Autodesk Fusion 360 part; units mm, degrees
sketch "Sketch1" plane through (0, 0, 0) normal (1, 0, 0) x (0, 1, 0)
sketch "Sketch2" plane through (0, 0, 0) normal (0, 0, 1) x (1, 0, 0)
sketch "Sketch3" plane through (0, 0, 0) normal (1, 0, 0) x (0, 1, 0)
sketch "Sketch4" plane through (0, 0, 0) normal (1, 0, 0) x (0, 1, 0)
sketch "Sketch5" plane through (0, 0, 0) normal (0, 1, 0) x (1, 0, 0)
  circle A0 centre (0, 0) radius 18
  circle A1 centre (0, 0) radius 8
  line L0 (0, 11.547) -> (-10, 5.7735)
  line L1 (-10, 5.7735) -> (-10, -5.7735)
  line L2 (-10, -5.7735) -> (0, -11.547)
  line L3 (0, -11.547) -> (10, -5.7735)
  line L4 (10, -5.7735) -> (10, 5.7735)
  line L5 (10, 5.7735) -> (0, 11.547)
  arc A2 (18.3848, -24.0416) -> (24.0416, -18.3848) centre (21.2132, -21.2132) ccw
  arc A3 (-18.3848, 24.0416) -> (-24.0416, 18.3848) centre (-21.2132, 21.2132) ccw
  line L6 (-21.2132, 21.2132) -> (21.2132, -21.2132) construction
  circle A4 centre (21.2132, -21.2132) radius 2
  circle A5 centre (-21.2132, 21.2132) radius 2
  arc A6 (24.0416, 18.3848) -> (18.3848, 24.0416) centre (21.2132, 21.2132) ccw
  arc A7 (-24.0416, -18.3848) -> (-18.3848, -24.0416) centre (-21.2132, -21.2132) ccw
  circle A8 centre (-21.2132, -21.2132) radius 2
  circle A9 centre (21.2132, 21.2132) radius 2
  arc A10 (24.0416, -24.0416) -> (24.0416, 24.0416) centre (0, 0) ccw
  arc A11 (24.0416, 24.0416) -> (-24.0416, 24.0416) centre (0, 0) ccw
  arc A12 (-24.0416, 24.0416) -> (-24.0416, -24.0416) centre (0, 0) ccw
  arc A13 (-24.0416, -24.0416) -> (24.0416, -24.0416) centre (0, 0) ccw
  line L7 (-24.0416, -18.3848) -> (-15.2381, -9.5812)
  line L8 (-21.2132, -21.2132) -> (-12.7279, -12.7279) construction
  line L9 (-9.5812, -15.2381) -> (-18.3848, -24.0416)
  line L10 (9.5812, -15.2381) -> (18.3848, -24.0416)
  line L11 (24.0416, -18.3848) -> (15.2381, -9.5812)
  line L12 (24.0416, 18.3848) -> (15.2381, 9.5812)
  line L13 (12.7279, 12.7279) -> (21.2132, 21.2132) construction
  line L14 (9.5812, 15.2381) -> (18.3848, 24.0416)
  line L15 (-9.5812, 15.2381) -> (-18.3848, 24.0416)
  line L16 (-24.0416, 18.3848) -> (-15.2381, 9.5812)
  line L17 (0, 0) -> (5.6569, 0) construction
  line L18 (8, 0) -> (30, 0) construction
  dimension "d3" = 36
  dimension "d4" = 16
  dimension "d5" = 10
  dimension "d8" = 8
  dimension "d9" = 45
  dimension "d10" = 4
  dimension "d11" = 4
  dimension "d12" = 60
  dimension "d14" = 34
  dimension "d16" = 360
sketch "Sketch6" plane through (0, 0, 0) normal (0, 1, 0) x (1, 0, 0)
extrude "Extrude1" add sketch "Sketch5" along normal blind 10 contours A0 | A0 A2 A6 A10 L11 L12 | A0 A6 L12 L14 | A0 A2 L10 L11 | A0 A3 A6 A11 L14 L15 | A0 A2 A7 A13 L9 L10 | A0 A3 L15 L16 | A0 A7 L7 L9 | A0 A3 A7 A12 L7 L16 | A1 | L0 L1 L2 L3 L4 L5
Can you work these out from the model? Positions are in its coordinate system, mm. Coordinates: 2 decimals unless noted, no trailing zeros. Loops run counter-clockwise (first coordinate to the right, second up) from the corner with the lowest first, then second, coordinate; pieces in that order, holes last. Notation, with made-up numbers: M 73,-13 L 123,-13 A31 ccw 123,25 Z; hole C -36,45 d4. An arc over 180 degrees is marked long. Return JSON: item names as keys, results as strings. Group by question number.
Item 1: If I drill on L1, parallel to X at y = 3.75, z = -21; L2, parallel to Z at x = 20, y = 8; L3, parallel to Z at x = -22, y = 6.75, over which ranges is the centre line in solid material (lowest first)? Write a range as from..to.
Item 2: Imagine slicing it at B-B (z = 13). Please give me the cut outline in (x, y).
Item 3: Thinking about a two-plate mould opening in X: for faces 1 (the flat face through (0, 10, 0)), 2 (the cylindrical face through (-19.3, 4.9, 21.8)), 3 (the cylindrical face through (33.708, 4.93, -4.45)), 4 (the cylindrical face through (23.12, 4.93, 21.81)), which applies, released by +X, released by -X, zero draft, split by the parting line, or undercut?
Item 4: I'm going to push flat-ended pins straight in: pin 1 Ø2 at (x, y) = (-26, 6.5) entering from +Z; pin 2 Ø3 at (x, y) = (-13.5, 2) entering from -Z; pin 3 Ø5 at (x, y) = (9.5, 7.5) entering from -Z. Where does each tip first touch, or does it pass through?
Item 5: Imagine slicing it at A-A (y = 3.5). Please give me the cut outline in (x, z), and give its area (3 significant figures).
Item 6: Imagine slicing it at C-C (x = 16). Please give me the cut outline in (y, z).
Verdict:
{
 "1": {"L1": "x = -26.74..-23.2, -19.22..19.22, 23.2..26.74", "L2": "z = -27.5..-22.8, -19.62..19.62, 22.8..27.5", "L3": "z = -25.92..-23.05, -19.37..19.37, 23.05..25.92"},
 "2": {"outline": "M -31.42,0 L 31.42,0 L 31.42,10 L -31.42,10 Z"},
 "3": {"face 1": "zero draft", "face 2": "undercut", "face 3": "split by the parting line", "face 4": "undercut"},
 "4": {"pin 1": "stops at z = 23.04", "pin 2": "stops at z = -31.81", "pin 3": "stops at z = -33.27"},
 "5": {"outline": "C 0,0 d68; hole C -21.21,-21.21 d4; hole C -21.21,21.21 d4; hole C 21.21,-21.21 d4; hole C 21.21,21.21 d4", "area": "3,580 mm^2"},
 "6": {"outline": "M 0,-30 L 10,-30 L 10,30 L 0,30 Z"}
}
